Input: part model. Units: mm. Frame: model coordinates. Give positions to 0.01 mm unless a question says otherwise; leave off trailing zeros. Loops run counter-clockwise (first coordinate to the right, second up) from the corner with the lowest first, then second, coordinate; pieces in that order, holes last. Notation, with made-up numbers: (81.5, 88) - (93.5, 88) arc R29 cw to (93.5, 123) - close; hole circle Ø4 at (5.5, 21). An arc over 180 degrees is marked (long way). Answer as a JSON object with one key per item and string values. Group by question number.
(1) Section query D-D (x = 7.25). Return loops of the section in (y, z), plus the area to 3 significant figures.
(2) Pin query (flat end, axial travel): P1, Ø2, axis at y = -5, z = 1.5, coming from the +X side; P2, Ø8, axis at x = 0, y = 1.5, coming from the +Z side. Return the tip coordinate at first contact, or that it passes through.
(3) Material intervals for L1, parallel to Y at x = 0, z = 2.25; L2, parallel to X at y = 2, z = -2.75; L3, parallel to Y at x = -5.75, z = -2.75, sorted ascending.
(4) Mould query, pull axis X, two halves, no side actions, for faces 1 (the cylindrical face through (-1.38, 6.2, -0.09)), 2 (the flat face through (7.396, -4.19, -0.089)), 3 (the flat face through (-7.396, 4.19, -0.089)), 4 (the flat face through (0, -8.5, 0)). Classes: +X half, -X half, draft (parallel to the pull), parting line (faces both ways), or undercut.
(5) Section query C-C (y = -4). Return loops of the section in (x, z).
(6) Section query A-A (x = 0). Return loops of the section in (y, z), plus the area to 3 significant figures.
Autodesk Inventor part; units mm, degrees
ref_plane "YZ Plane" through (0, 0, 0) normal (1, 0, 0) x (0, 1, 0)
ref_plane "XZ Plane" through (0, 0, 0) normal (0, 1, 0) x (-1, 0, 0)
ref_plane "XY Plane" through (0, 0, 0) normal (0, 0, 1) x (1, 0, 0)
sketch "Sketch1" plane through (0, 0, 0) normal (0, 0, 1) x (1, 0, 0)
  line L0 (4.9075, 8.5) -> (9.815, 0)
  line L1 (9.815, 0) -> (4.9075, -8.5)
  line L2 (4.9075, -8.5) -> (-4.9075, -8.5)
  line L3 (-4.9075, -8.5) -> (-9.815, 0)
  line L4 (-9.815, 0) -> (-4.9075, 8.5)
  line L5 (-4.9075, 8.5) -> (4.9075, 8.5)
  circle A0 centre (0, 0) radius 6.35
  dimension "d0" = 17
  dimension "d1" = 12.7
extrude "Extrusion1" add sketch "Sketch1" along normal mid plane 12.7
equation "\"d0\" = hexOutput"
equation "\"d1\" = shaftSize"
equation "\"d2\" = length"
equation "\"hexOutput\" = 17"
equation "\"shaftSize\" = 12.7"
equation "\"length\" = 12.7"
properties part number "17mmTo0.5inchBearing"
Recorded:
{
 "1": {"outline": "(-4.44, -6.35) - (4.44, -6.35) - (4.44, 6.35) - (-4.44, 6.35) - close", "area": "113 mm^2"},
 "2": {"P1": "stops at x = 7.51", "P2": "passes through"},
 "3": {"L1": "y = -8.5 to -6.35, 6.35 to 8.5", "L2": "x = -8.66 to -6.03, 6.03 to 8.66", "L3": "y = -7.04 to -2.69, 2.69 to 7.04"},
 "4": {"face 1": "undercut", "face 2": "+X half", "face 3": "-X half", "face 4": "draft"},
 "5": {"outline": "(-7.51, -6.35) - (-4.93, -6.35) - (-4.93, 6.35) - (-7.51, 6.35) - close; (4.93, -6.35) - (7.51, -6.35) - (7.51, 6.35) - (4.93, 6.35) - close"},
 "6": {"outline": "(-8.5, -6.35) - (-6.35, -6.35) - (-6.35, 6.35) - (-8.5, 6.35) - close; (6.35, -6.35) - (8.5, -6.35) - (8.5, 6.35) - (6.35, 6.35) - close", "area": "54.6 mm^2"}
}
